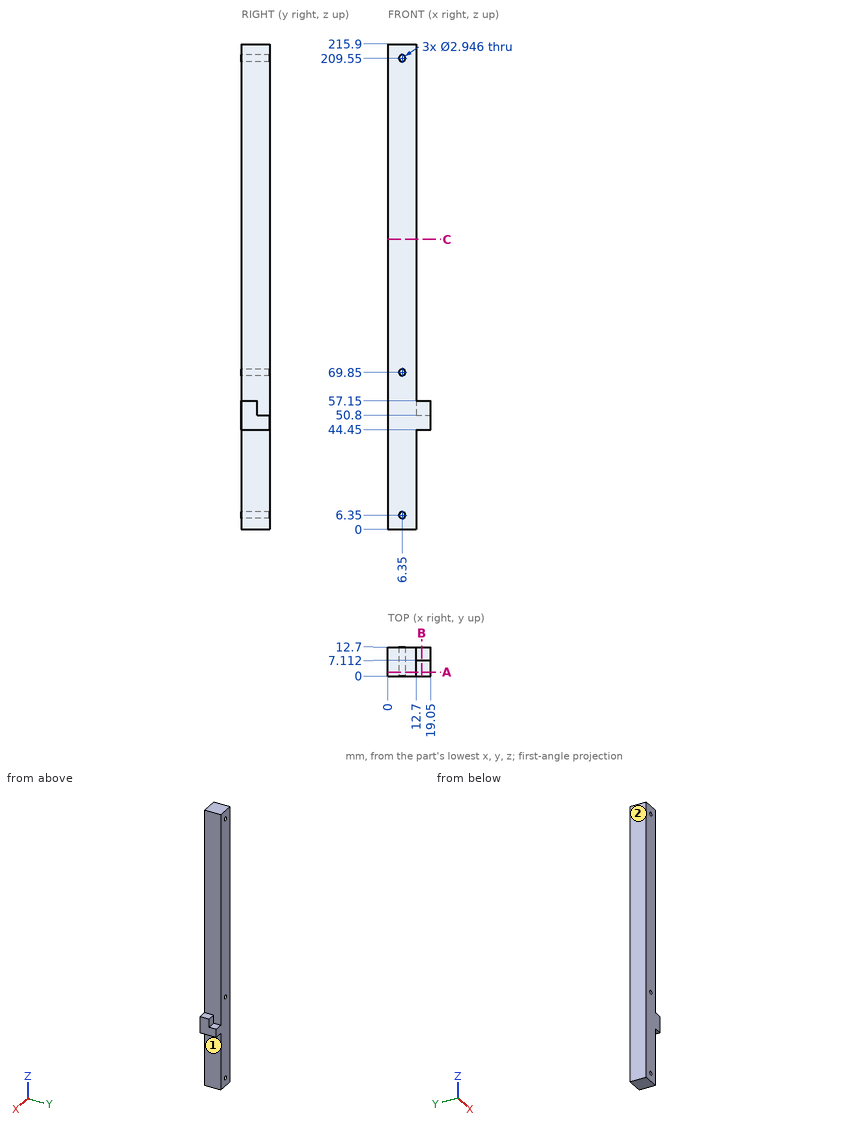
Could you check a few things on this drawing? It's one solid part, dimensions in mm from its lowest x, y, z. A direction names the side the tool comes from. Round coordinates to 2 decimals unless told otherwise and drop trailing zeros. Write each loop counter-clockwise with the first axis right and the second up, starting at its lowest first coordinate (ties: lowest second). Pieces come first, ordered by that corner, then holes.
Q1. Will these pins go through, and if not, where does the flat tip stop? P1, Ø1.9, axis at x = 17, y = 4.5, coming from the +Z side; P2, Ø3, axis at x = 15.5, y = 9, coming from the -Z side; P3, Ø3, axis at x = 15, y = 11, coming from the +Z side.
Q2. If we section it at A-A on y = 1.75: Write out the boundary of the cut face in (x, z).
Q3. Please list where these lines run through material, in increasing order: probe 1 along Z at (x, y) = (6.35, 9.75); probe 2 along X at (y, z) = (5, 209.55); probe 3 along Z at (x, y) = (14, 10.5).
Q4. If we section it at C-C on z = 129: Write out the boundary of the cut face in (x, y), plus the area to 3 significant figures.
Q5. Which directions (+Z, -Z, +X, -X, +Y, -Y) give clear straight access to the entire face, cutting with the end or side of a thin tool? Please do the marked faces 1 and 2.
Q6. If we section it at B-B on x = 15: Write out the boundary of the cut face in (y, z), plus the area to 3 significant figures.
Answer below:
1. P1: stops at z = 57.15
1. P2: stops at z = 44.45
1. P3: stops at z = 50.8
2. outline: (0, 0) - (12.7, 0) - (12.7, 44.45) - (19.05, 44.45) - (19.05, 57.15) - (12.7, 57.15) - (12.7, 215.9) - (0, 215.9) - close; hole circle Ø2.95 at (6.35, 6.35); hole circle Ø2.95 at (6.35, 69.85); hole circle Ø2.95 at (6.35, 209.55)
3. probe 1: z = 0 to 4.88, 7.82 to 68.38, 71.32 to 208.08, 211.02 to 215.9
3. probe 2: x = 0 to 4.88, 7.82 to 12.7
3. probe 3: z = 44.45 to 50.8
4. outline: (0, 0) - (12.7, 0) - (12.7, 12.7) - (0, 12.7) - close
4. area: 161 mm2
5. face 1: -Z, +X, +Y, -Y
5. face 2: +Z, -Z, -X, +Y, -Y
6. outline: (0, 44.45) - (12.7, 44.45) - (12.7, 50.8) - (7.11, 50.8) - (7.11, 57.15) - (0, 57.15) - close
6. area: 126 mm2
